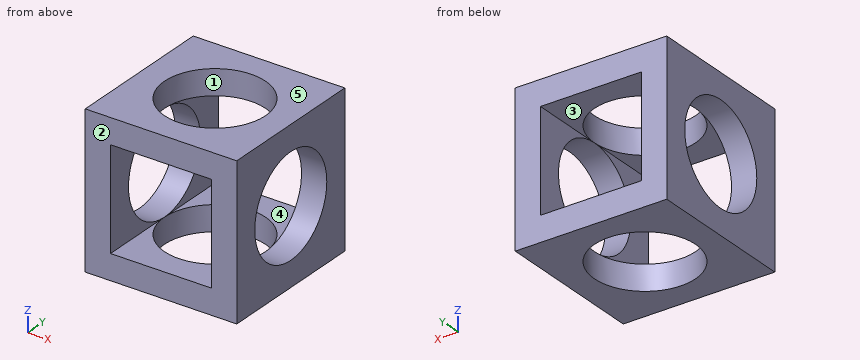
from build123d import *

# Parameters (mm, degrees)
F0_W      = 30
F0_H      = 30
F1_DEPTH  = 15
F1_FACE_W = 30
F1_FACE_H = 30
F2_DEPTH  = 15
F3_W      = 20
F3_H      = 20
F4_DEPTH  = 30.001
F5_R      = 10
F6_DEPTH  = 30.001
F7_R      = 10
F8_DEPTH  = 30.001


with BuildPart() as f1:
    # F0 (on Front) → F1 (new body)
    with BuildSketch(Plane.XZ):
        Rectangle(F0_W, F0_H)
    extrude(amount=F1_DEPTH)

    # F1_face (on face) → F2 (join)
    with BuildSketch(Plane(origin=(0, 0, 0), x_dir=(1, 0, 0), z_dir=(0, 1, 0))):
        Rectangle(F1_FACE_W, F1_FACE_H)
    extrude(amount=F2_DEPTH)

    # F3 (on face) → F4 (cut, through all)
    with BuildSketch(Plane.XZ.offset(15)):
        Rectangle(F3_W, F3_H)
    extrude(amount=-F4_DEPTH, mode=Mode.SUBTRACT)

    # F5 (on face) → F6 (cut, through all)
    with BuildSketch(Plane.XY.offset(15)):
        Circle(F5_R)
    extrude(amount=-F6_DEPTH, mode=Mode.SUBTRACT)

    # F7 (on face) → F8 (cut, through all)
    with BuildSketch(Plane(origin=(-15, 0, 0), x_dir=(0, -1, 0), z_dir=(-1, 0, 0))):
        Circle(F7_R)
    extrude(amount=-F8_DEPTH, mode=Mode.SUBTRACT)


solid = f1.part
Can you work these out from the model? Positions are in its coordinate system, mm. Face numbers are marked on the shaded views. A direction names the side the tool comes from. Give positions to 0.01 mm unless a question says otherwise; leave off trailing zeros. Write each loop counter-clockwise with the first axis right and the second up, starting at its lowest first coordinate (ties: lowest second). Pieces come first, ordered by that corner, then holes. Notation, with made-up numbers: (-17.5, 64) -> (5.5, 64) arc R21 cw to (5.5, 87) -> close; hole circle Ø3 at (70, 45.25). An arc over 180 degrees is marked (long way). Answer as a JSON object with one key per item and string values. Group by question number.
Item 1: Suppose I cut it at A-A (x = 0). Please give me the cut outline in (y, z), plus the area to 3 significant figures.
Item 2: Please list where this line runs through material, in increasing order: line 1 (Y direction, x = 0, z = -12.35). Write a range as [from, to].
Item 3: Suppose I cut it at D-D (z = 10.75). Please give me the cut outline in (x, y).
Item 4: We'd pull the mould along Y, two halves only. Please class the marked faces 1, 2 and 3: +Y half, -Y half, draft (parallel to the pull), parting line (faces both ways), or undercut.
Item 5: Suppose I cut it at C-C (y = 11). Please give me the cut outline in (x, z), plus the area to 3 significant figures.
Item 6: I'm going to push a flat-ended pin straight in: P1, Ø4.5, axis at y = -5.5, z = -4, coming from the -X side. Where does the tip first touch, or does it pass through?
Item 7: For the marked faces 4 and 5, which set-ups out of +Z, -Z, +X, -X, +Y, -Y let a thin tool reach every point of the face, with its end or its side?
Findings:
{
 "1": {"outline": "(-15, -15) -> (-10, -15) -> (-10, -10) -> (-15, -10) -> close; (-15, 10) -> (-10, 10) -> (-10, 15) -> (-15, 15) -> close; (10, -15) -> (15, -15) -> (15, -10) -> (10, -10) -> close; (10, 10) -> (15, 10) -> (15, 15) -> (10, 15) -> close", "area": "100 mm²"},
 "2": {"line 1": "y = [-15, -10], [10, 15]"},
 "3": {"outline": "(-15, -15) -> (15, -15) -> (15, 15) -> (-15, 15) -> close; hole circle Ø20 at (0, 0)"},
 "4": {"face 1": "undercut", "face 2": "-Y half", "face 3": "draft"},
 "5": {"outline": "(-15, -15) -> (15, -15) -> (15, 15) -> (-15, 15) -> close; hole (-10, -10) -> (10, -10) -> (10, 10) -> (-10, 10) -> close", "area": "500 mm²"},
 "6": {"P1": "passes through"},
 "7": {"face 4": "+Y, -Y", "face 5": "+Z, +X, -X, +Y, -Y"}
}
